Can you work these out from the model? Positions are in its coordinate system, mm. A direction names the side the tool comes from. Coordinates: 2 decimals unless noted, no trailing zeros. Loops run counter-clockwise (first coordinate to the right, second up) from the corner with the lowest first, then second, coordinate; pieces in that order, holes last. Notation, with made-up numbers: (29.5, 57) -> (46.5, 57) arc R38 cw to (46.5, 95) -> close; hole circle Ø5 at (9, -7.5). An arc over 180 degrees is marked (long way). Put each result on its own line as item: value. Start each with the question number.
Item 1: If we section it at B-B on z = -2: Please give me the cut outline in (x, y), plus the area to 3 significant figures.
Item 2: Will these pins go through, and if not, where does the flat tip stop? P1, Ø18, axis at y = -79, z = -18.5, coming from the +X side; P2, Ø6.5, axis at x = 0, y = -87.3, coming from the +Z side; P3, Ø10, axis at x = 0.5, y = -83.5, coming from the -Z side; P4, Ø3.5, axis at x = 0, y = -67.3, coming from the +Z side.
Item 3: If we section it at D-D on x = 13: Please give me the cut outline in (y, z).
Item 4: Please list where these lines run through material, in increasing order: L1, parallel to Z at x = 12.05, y = -90.05; L2, parallel to Y at x = 0, z = 0.8; L3, parallel to Z at x = 20.5, y = -78. Write a range as from..to.
Item 5: We'd pull the mould along Z, two halves only. Please class faces 1 (the cylindrical face through (18.002, -72.44, -0.336)), 2 (the flat face through (16.869, -72.44, 4.375)), 3 (the cylindrical face through (25.745, -77.37, -0.225)): pulls with the +Z half, pulls with the -Z half, needs draft (parallel to the pull), parting line crosses it, or undercut.
Item 6: For faces 4 (the flat face through (0, -77, 0)), 5 (the flat face through (2, -77, 4)), 6 (the flat face through (17, -72, -5.696)), which set-ups out of +Z, -Z, +X, -X, +Y, -Y let a thin tool reach every point of the face, with its end or its side?
Item 7: If we section it at A-A on x = 0: Please give me the cut outline in (y, z).
Autodesk Inventor part; units mm, degrees
ref_plane "Work Plane1" through (-10, -77.3, 0) normal (0, 1, 0) x (1, 0, 0)
ref_plane "YZ Plane" through (0, 0, 0) normal (1, 0, 0) x (0, 1, 0)
ref_plane "XZ Plane" through (0, 0, 0) normal (0, 1, 0) x (-1, 0, 0)
sketch "Sketch1" plane through (0, 0, 0) normal (0, 0, 1) x (1, 0, 0)
  line L0 (10, 0) -> (10, -500)
  line L1 (-10, 0) -> (-10, -500)
  line L2 (13.8571, -62.3) -> (-6.0929, -62.3)
  line L3 (10, -62.3) -> (-10, -62.3)
  line L4 (-10, -62.3) -> (-10, -92.3)
  line L5 (-10, -92.3) -> (10, -92.3)
  line L6 (10, -92.3) -> (10, -62.3)
  circle A0 centre (0, -87.3) radius 2
  circle A1 centre (0, -67.3) radius 2
  point P0 (0, 0)
  dimension "d0" = 30
  dimension "d1" = 4
  dimension "d2" = 4
  dimension "d3" = 5
  dimension "d4" = 5
extrude "Extrusion1" add sketch "Sketch1" along normal blind 4
ref_plane "Work Plane1" through (-10, -77.3, 0) normal (0, 1, 0) x (1, 0, 0)
sketch "Sketch3" plane through (10, -92.3, 0) normal (1, 0, 0) x (0, 0, -1)
  line L0 (0, 0) -> (0, 30)
  line L1 (0, 30) -> (-4, 30)
  line L2 (-4, 0) -> (-4, 30)
  line L3 (0, 0) -> (-4, 0)
  line L4 (0, 0) -> (0, 30)
  line L5 (0, 0) -> (20, 0)
  line L6 (20, 0) -> (20, 30)
  line L7 (20, 30) -> (0, 30)
  line L8 (0, 30) -> (0, 0)
  circle A0 centre (10, 25) radius 2
  circle A1 centre (10, 5) radius 2
  point P0 (0, 92.3)
  dimension "d12" = 20
  dimension "d13" = 4
  dimension "d14" = 4
  dimension "d15" = 5
  dimension "d16" = 5
extrude "Extrusion3" add sketch "Sketch3" along normal blind 4 contours L3 L2 L1 L0 | L0 L7 L6 L5 | A0 | A1
sketch "Sketch2" plane through (-10, -77.3, 0) normal (0, 1, 0) x (1, 0, 0)
  line L0 (20, -4) -> (0, -4)
  line L1 (20, 0) -> (0, 0)
  line L2 (0, 0) -> (0, -4)
  line L3 (0, -4) -> (24, -4)
  line L4 (24, 20) -> (24, -4)
  line L5 (20, 20) -> (24, 20)
  line L6 (20, 20) -> (20, 0)
  line L7 (24, -4) -> (24, 20)
  circle A0 centre (30.5, 0.4456) radius 2.5
  circle A1 centre (30.5, 0.4456) radius 5.25
  line L8 (24, 20) -> (34.8957, 3.3163)
  line L9 (24, -4) -> (29.82, -4.7602)
  line L10 (30.5, 5.6956) -> (24, 5.6956)
  point P0 (10, 0)
  point P1 (24, 0.4456)
  dimension "d26" = 5
  dimension "d27" = 2.75
  dimension "d29" = 4.4456
  dimension "d30" = 6.5
  dimension "d50" = 10.5
extrude "Extrusion2" add sketch "Sketch2" along normal mid plane 10 contours L4 L10 A1 L9 | A1
sketch "Sketch4" plane through (-10, -72.3, 0) normal (0, 1, 0) x (1, 0, 0)
  line L0 (23.958, -4) -> (24, -4)
  line L1 (24, -4) -> (24, -8.9113)
  arc A0 (29.82, -4.7602) -> (30.5, 5.6956) centre (30.5, 0.4456) ccw
  circle A1 centre (30.5, 0.4456) radius 2.5
  line L2 (30.5, 5.6956) -> (24, 5.6956)
  line L3 (24, -4) -> (24, 5.6956)
  line L4 (24, -4) -> (29.82, -4.7602)
  point P0 (10, 0)
  point P1 (0, -4)
  point P2 (24, -4.0444)
extrude "Extrusion4" add sketch "Sketch4" along normal blind 10
fillet "Fillet1" [suppressed]
sketch "Sketch5" plane through (-10, -62.3, 4) normal (0, 1, 0) x (1, 0, 0)
  circle A0 centre (30.5, 4.4456) radius 2.5
  line L0 (20, 24) -> (22, 44)
  line L1 (22, 44) -> (24, 44)
  line L2 (24, 44) -> (21.9516, 23.5162)
  line L3 (20, 24) -> (24, 24)
  point P0 (10, 4)
  point P1 (22, 24)
  dimension "d38" = 2
  dimension "d39" = 6.5
  dimension "d40" = 20
extrude "Extrusion5" [suppressed]
fillet "Fillet2" [suppressed]
sketch "Sketch6" plane through (0, 0, 4) normal (0, 0, 1) x (1, 0, 0)
  circle A0 centre (14, -64.8) radius 2.1
  line L0 (25.7065, -62.3) -> (14, -62.3)
  line L1 (10, -92.3) -> (10, -62.3)
  line L2 (18, -62.3) -> (18, -82.3)
  line L3 (23, -62.3) -> (23, -96.3)
  line L4 (19.3, -67.6) -> (49.3, -67.6)
  line L5 (19.45, -67.3) -> (49.45, -67.3)
  point P0 (0, 0)
  dimension "d42" = 4.2
  dimension "d43" = 2.5
  dimension "d44" = 4
extrude "Extrusion6" cut sketch "Sketch6" along normal mid plane 100
chamfer "Chamfer1" distance 3 distance2 2 1 edges at (14, -92.3, -8) measured on face at (14, -80.5, -15.2319)
sketch "Sketch7" plane through (10, -92.3, -20) normal (0, 0, -1) x (-1, 0, 0)
  line L0 (-2, 0) -> (-4, 3)
  line L1 (0, 0) -> (-2, 0)
  line L2 (0, 0) -> (0, 30)
  line L3 (0, 30) -> (-4, 30)
  line L4 (-4, 29.6) -> (-4, 30)
  arc A0 (-4, 25.4) -> (-4, 29.6) centre (-4, 27.5) ccw
  line L5 (-4, 3) -> (-4, 25.4)
  point P0 (10, 92.3)
extrude "Extrusion7" add sketch "Sketch7" along normal blind 20
sketch "Sketch8" plane through (14, -92.3, 0) normal (1, 0, 0) x (0, 0, -1)
  line L0 (2.9456, 30) -> (2.9456, 10)
  line L1 (-2.0544, 30) -> (-2.0544, 10)
  circle A0 centre (23.9956, 2.25) radius 12
  line L2 (5.6956, 10) -> (-4, 10)
  point P0 (0, 92.3)
  point P1 (0.4456, 12.1254)
  dimension "d53" = 5
  dimension "d54" = 2.5
  dimension "d55" = 24
  dimension "d56" = 7.75
  dimension "d57" = 23.55
extrude "Extrusion8" cut sketch "Sketch8" against normal blind 10
fillet "Fillet3" radius 2 2 edges at (10, -78.05, -23.9956) (14, -78.05, -23.9956)
equation "\"d16\" = d15"
equation "\"d7\" = -0.5 * d0"
properties part number "tool dock" material "Polycarbonate, Clear"
Solutions:
1. outline: (10, -92.3) -> (12, -92.3) -> (14, -89.3) -> (14, -82.3) -> (18.54, -82.3) -> (18.54, -62.3) -> (10, -62.3) -> close; (22.46, -82.3) -> (25.51, -82.3) -> (25.51, -62.3) -> (22.46, -62.3) -> close; hole circle Ø4.2 at (14, -64.8)
1. area: 255 mm^2
2. P1: x = 14
2. P2: z = 4
2. P3: z = 0
2. P4: through
3. outline: (-90.8, -40) -> (-66.65, -40) -> (-66.65, 4) -> (-90.8, 4) -> (-90.8, -11.75) arc R12.27 cw (long way) to (-90.8, -36.24) -> close; (-62.95, -40) -> (-62.3, -40) -> (-62.3, 4) -> (-62.95, 4) -> close
4. L1: -40..-36, -11.99..4
4. L2: -92.3..-89.3, -85.3..-69.3, -65.3..-62.3
4. L3: -5.7..-2.95, 2.05..4.8
5. face 1: undercut
5. face 2: pulls with the +Z half
5. face 3: parting line crosses it
6. face 4: -Z, -X, +Y, -Y
6. face 5: +Z, -X, +Y, -Y
6. face 6: -Z, +X, +Y, -Y
7. outline: (-92.3, 0) -> (-89.3, 0) -> (-89.3, 4) -> (-92.3, 4) -> close; (-85.3, 0) -> (-69.3, 0) -> (-69.3, 4) -> (-85.3, 4) -> close; (-65.3, 0) -> (-62.3, 0) -> (-62.3, 4) -> (-65.3, 4) -> close
